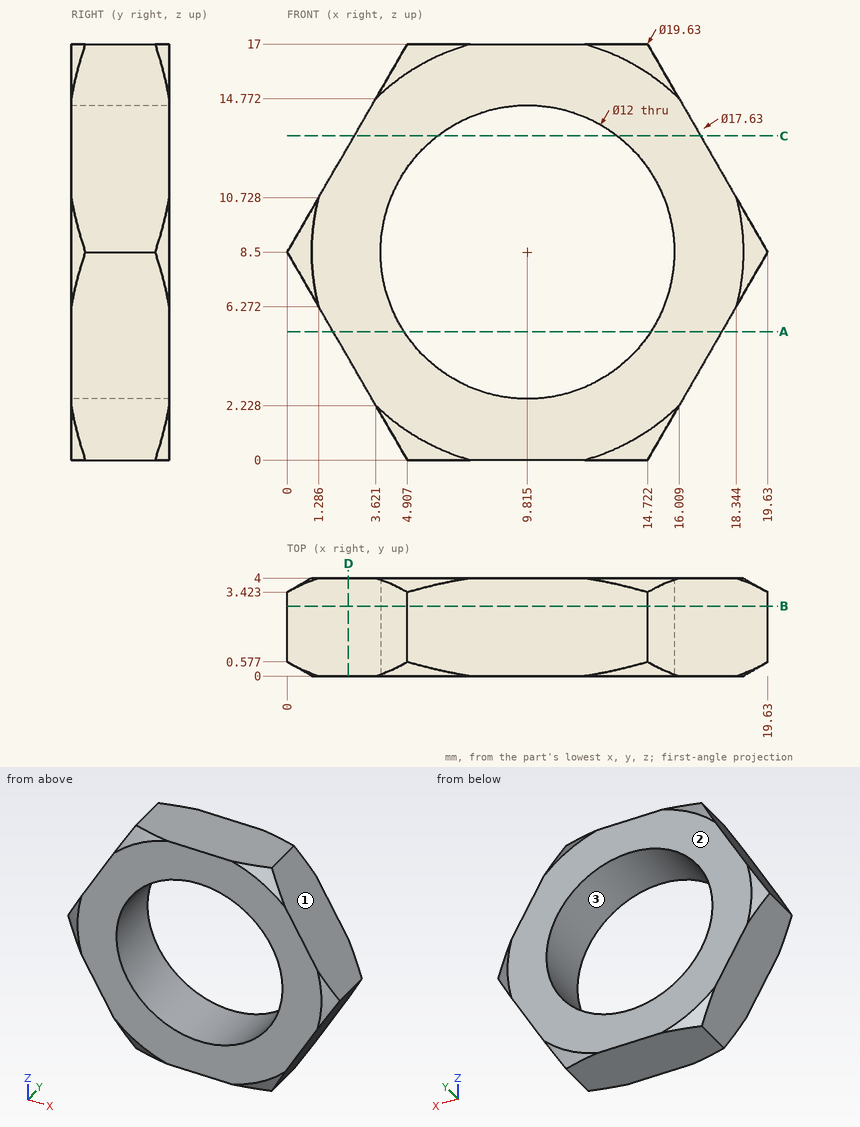
Verification items for this drawing (mm, ordinates from the low corner). Coordinates: 2 decimals unless noted, no trailing zeros. Loops run counter-clockwise (first coordinate to the right, second up) from the corner with the lowest first, then second, coordinate; pieces in that order, holes last.
Item 1: Thickness scan on line 1 (Z direction, x = 8, y = 2.6); line 2 (X direction, y = 2.15, z = 12.5) (1 decimal); line 3 (X direction, y = 2.75, z = 8.75) (1 decimal). Record the ranges inside material, lowest first.
Item 2: Go/stop test with a flat-tipped pin: pin 1 Ø2 at (y, z) = (0.5, 13.5) entering from -X. Record where the tip stops, or that it passes through.
Item 3: Sectioned sample at B-B, the plane y = 2.85. Record the boundary of the cut face in (x, z) (1 decimal), then the cut area to 3 significant figures.
Item 4: Release check for a two-part mould opening along X. For the marked faces 1, 2 and 3 record: released by +X, released by -X, zero draft, split by the parting line, or undercut.
Item 5: Sectioned sample at C-C, the plane z = 13.25. Record the boundary of the cut face in (x, y).
Item 6: Sectioned sample at A-A, the plane z = 5.25. Record the boundary of the cut face in (x, y).
Item 7: Sectioned sample at D-D, the plane x = 2.5. Record the boundary of the cut face in (y, z).
Check result:
1. line 1: z = 0 to 2.78, 14.22 to 17
1. line 2: x = 2.3 to 5.3, 14.3 to 17.3
1. line 3: x = 0.1 to 3.8, 15.8 to 19.5
2. pin 1: stops at x = 2.31
3. outline: (0, 8.5) - (4.9, 0) - (14.7, 0) - (19.6, 8.5) - (14.7, 17) - (4.9, 17) - close; hole circle Ø12 at (9.8, 8.5)
3. area: 137 mm2
4. face 1: released by +X
4. face 2: zero draft
4. face 3: undercut
5. outline: (2.74, 0) - (6.15, 0) - (6.15, 4) - (2.74, 4) - close; (13.48, 0) - (16.89, 0) - (16.89, 4) - (13.48, 4) - close
6. outline: (1.88, 0) - (4.77, 0) - (4.77, 4) - (1.88, 4) - close; (14.86, 0) - (17.75, 0) - (17.75, 4) - (14.86, 4) - close
7. outline: (0, 4.17) - (4, 4.17) - (4, 12.83) - (0, 12.83) - close
